The model under review builds one solid part; all positions refer to its coordinate system, in mm. Face numbers are marked on the shaded views. A direction names the side the tool comes from. Give positions to 0.01 mm unless a question says otherwise; leave off trailing zeros. Order: outer loops, then holes, each group sorted by start corner. A loop starts at its lowest first (then second) coordinate and runs counter-clockwise, first axis right, second up. Notation, with made-up numbers: (0.5, 16.25) - (25.5, 16.25) arc R9 cw to (25.5, 33.25) - close; hole circle Ø5 at (40.5, 50.5). An arc over 180 degrees is marked (long way). Write item = value, one per line. Start each with the question number.
1. We need section D-D, the plane z = 19.5. Give the boundary of the cut face in (x, y).
2. Wall thickness on probe 1 along X at (y, z) = (3.5, 29.5); probe 2 along Z at (x, y) = (6, 5.5); probe 3 along Z at (x, y) = (-6, 5.75): over which ranges is each line inside the solid? List them lowest first.
3. We need section B-B, the plane y = -3.5. Give the boundary of the cut face in (x, z) (3 decimals), and give its area (3 significant figures).
4. We need section C-C, the plane x = -5. Give the boundary of the cut face in (y, z).
5. Machinability: for the marked faces 1, 2 and 3, which of the approach directions +Z, -Z, +X, -X, +Y, -Y give a long, thin tool a straight path to every point of the face, cutting with its end or side? Answer none if there is none.
6. For P1, Ø6, axis at x = -13.5, z = 23.93, coming from the -Y side; P2, Ø4, axis at x = 1.86, z = 23.93, coming from the -Y side; P3, Ø1.4, axis at x = 2.5, z = 23.5, coming from the +Y side, all flat-tipped, find the tip position at first contact; note any pin that passes through.
7. We need section A-A, the plane y = 3. Give the boundary of the cut face in (x, z) (1 decimal), and give its area (3 significant figures).
8. Mouldability with a two-part tool opening along X and no side actions: class the marked faces 4, 5, 6 and 7 as pulls with the +X half, pulls with the -X half, needs draft (parallel to the pull), parting line crosses it, or undercut.
from build123d import *

# Parameters (mm, degrees)
F0_W          = 31.83
F0_H          = 15.82
F0_R          = 2.435
F1_DEPTH      = 2.5
F1_DEPTH_BACK = 9.6
F2_DEPTH      = 5
F3_R          = 3.215
F3_R_2        = 2.385
F4_DEPTH      = 8.4


with BuildPart() as f1:
    # F0 (on Front) → F1 (new body, two sides)
    with BuildSketch(Plane.XZ) as f1_sk:
        with Locations((-5.828721876, 24.0466938629)):
            Rectangle(F0_W, F0_H)
        with Locations((-17.828721876, 20.0516938629)):
            Circle(F0_R, mode=Mode.SUBTRACT)
        with Locations((-9.858721876, 20.0516938629)):
            Circle(F0_R, mode=Mode.SUBTRACT)
        with Locations((-1.798721876, 20.0516938629)):
            Circle(F0_R, mode=Mode.SUBTRACT)
        with Locations((6.171278124, 20.0516938629)):
            Circle(F0_R, mode=Mode.SUBTRACT)
        with Locations((-17.828721876, 28.0416938629)):
            Circle(F0_R, mode=Mode.SUBTRACT)
        with Locations((-9.858721876, 28.0416938629)):
            Circle(F0_R, mode=Mode.SUBTRACT)
        with Locations((-1.798721876, 28.0416938629)):
            Circle(F0_R, mode=Mode.SUBTRACT)
        with Locations((6.171278124, 28.0416938629)):
            Circle(F0_R, mode=Mode.SUBTRACT)
        with Locations((-1.798721876, 28.0416938629)):
            Circle(F0_R)
        with Locations((-9.858721876, 28.0416938629)):
            Circle(F0_R)
        with Locations((-17.828721876, 28.0416938629)):
            Circle(F0_R)
        with Locations((-17.828721876, 20.0516938629)):
            Circle(F0_R)
        with Locations((-9.858721876, 20.0516938629)):
            Circle(F0_R)
        with Locations((-1.798721876, 20.0516938629)):
            Circle(F0_R)
        with Locations((6.171278124, 20.0516938629)):
            Circle(F0_R)
        with Locations((6.171278124, 28.0416938629)):
            Circle(F0_R)
    extrude(amount=F1_DEPTH)
    extrude(f1_sk.sketch, amount=-F1_DEPTH_BACK)

    # F0 (on Front) → F2 (join)
    with BuildSketch(Plane.XZ):
        with Locations((-17.828721876, 28.0416938629)):
            Circle(F0_R)
        with Locations((-17.828721876, 20.0516938629)):
            Circle(F0_R)
        with Locations((-9.858721876, 28.0416938629)):
            Circle(F0_R)
        with Locations((-9.858721876, 20.0516938629)):
            Circle(F0_R)
        with Locations((-1.798721876, 28.0416938629)):
            Circle(F0_R)
        with Locations((-1.798721876, 20.0516938629)):
            Circle(F0_R)
        with Locations((6.171278124, 28.0416938629)):
            Circle(F0_R)
        with Locations((6.171278124, 20.0516938629)):
            Circle(F0_R)
    extrude(amount=F2_DEPTH)

    # F3 (on face) → F4 (cut)
    with BuildSketch(Plane(origin=(0, 9.6, 0), x_dir=(-1, 0, 0), z_dir=(0, 1, 0))):
        with BuildLine():
            Line((5.4793441668, 30.6818692116), (-8.7347330976, 30.6818692116))
            Line((-8.7347330976, 30.6818692116), (-8.7347330976, 17.3618692116))
            Line((-8.7347330976, 17.3618692116), (5.4793441668, 17.3618692116))
            Line((5.4793441668, 17.3618692116), (5.4793441668, 20.733492265))
            ThreePointArc((5.4793441668, 20.733492265), (2.6052669024, 23.9303652197), (5.4793441668, 27.1272381744))
            Line((5.4793441668, 27.1272381744), (5.4793441668, 30.6818692116))
        make_face()
        with Locations((-1.8597330976, 23.9303652197)):
            Circle(F3_R, mode=Mode.SUBTRACT)
        with BuildLine():
            Line((6.6202669024, 30.6818692116), (6.2793441668, 30.6818692116))
            Line((6.2793441668, 30.6818692116), (6.2793441668, 27.1124200692))
            ThreePointArc((6.2793441668, 27.1124200692), (8.2505095246, 26.0351563727), (9.0352669024, 23.9303652197))
            ThreePointArc((9.0352669024, 23.9303652197), (8.2505095246, 21.8255740668), (6.2793441668, 20.7483103702))
            Line((6.2793441668, 20.7483103702), (6.2793441668, 17.3618692116))
            Line((6.2793441668, 17.3618692116), (6.6202669024, 17.3618692116))
            Line((6.6202669024, 17.3618692116), (20.3752669024, 17.3618692116))
            Line((20.3752669024, 17.3618692116), (20.3752669024, 30.6818692116))
            Line((20.3752669024, 30.6818692116), (6.6202669024, 30.6818692116))
        make_face()
        with Locations((13.5002669024, 23.9303652197)):
            Circle(F3_R, mode=Mode.SUBTRACT)
        with Locations((-1.8597330976, 23.9303652197)):
            Circle(F3_R_2)
        with Locations((13.5002669024, 23.9303652197)):
            Circle(F3_R_2)
        with BuildLine():
            Line((5.4793441668, 21.5698575014), (5.4793441668, 26.290872938))
            ThreePointArc((5.4793441668, 26.290872938), (3.4352669024, 23.9303652197), (5.4793441668, 21.5698575014))
        make_face()
        with BuildLine():
            ThreePointArc((8.2052669024, 23.9303652197), (7.6618863359, 25.4458396874), (6.2793441668, 26.2707654131))
            Line((6.2793441668, 26.2707654131), (6.2793441668, 21.5899650263))
            ThreePointArc((6.2793441668, 21.5899650263), (7.6618863359, 22.414890752), (8.2052669024, 23.9303652197))
        make_face()
        with BuildLine():
            ThreePointArc((6.2793441668, 26.2707654131), (5.8801935351, 26.3146122285), (5.4793441668, 26.290872938))
            Line((5.4793441668, 26.290872938), (5.4793441668, 21.5698575014))
            ThreePointArc((5.4793441668, 21.5698575014), (5.8801935351, 21.546118211), (6.2793441668, 21.5899650263))
            Line((6.2793441668, 21.5899650263), (6.2793441668, 26.2707654131))
        make_face()
    extrude(amount=-F4_DEPTH, mode=Mode.SUBTRACT)


solid = f1.part
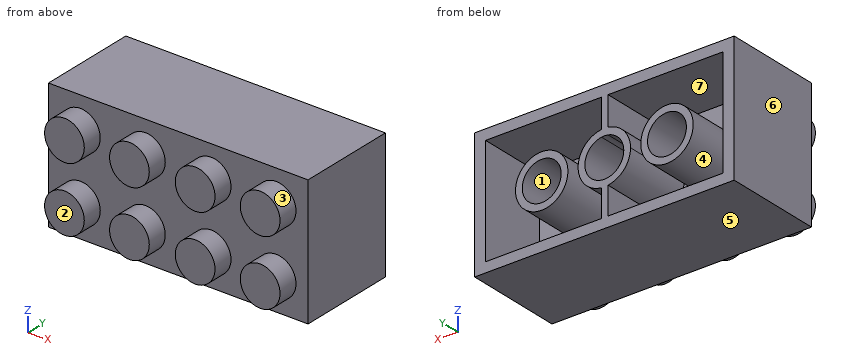
Model answer:
q1.outline = (-21.74, -2.5) - (-20.2, -2.5) - (-20.2, -5) - (-15.46, -5) - (-15.46, -2.5) - (-12.23, -2.5) - (-12.23, -5) - (-7.49, -5) - (-7.49, -2.5) - (-4.17, -2.5) - (-4.17, -5) - (0.57, -5) - (0.57, -2.5) - (3.8, -2.5) - (3.8, -5) - (8.54, -5) - (8.54, -2.5) - (10.09, -2.5) - (10.09, 9.6) - (8.73, 9.6) - (8.73, 1.2) - (-5.48, 1.2) - (-5.48, 9.6) - (-6.28, 9.6) - (-6.28, 1.2) - (-20.38, 1.2) - (-20.38, 9.6) - (-21.74, 9.6) - close
q2.probe_1 = -21.74 to -20.38, -6.28 to -5.48, 8.73 to 10.09
q2.probe_2 = 16.14 to 17.36, 30.68 to 31.96
q2.probe_3 = 16.14 to 21.55, 26.31 to 31.96
q3.outline = circle Ø4.87 at (-17.829, 20.052); circle Ø4.87 at (-17.829, 28.042); circle Ø4.87 at (-9.859, 20.052); circle Ø4.87 at (-9.859, 28.042); circle Ø4.87 at (-1.799, 20.052); circle Ø4.87 at (-1.799, 28.042); circle Ø4.87 at (6.171, 20.052); circle Ø4.87 at (6.171, 28.042)
q3.area = 149 mm2
q4.outline = (-2.5, 16.14) - (9.6, 16.14) - (9.6, 17.36) - (1.2, 17.36) - (1.2, 20.82) - (9.6, 20.82) - (9.6, 21.69) - (1.2, 21.69) - (1.2, 26.17) - (9.6, 26.17) - (9.6, 27.04) - (1.2, 27.04) - (1.2, 30.68) - (9.6, 30.68) - (9.6, 31.96) - (-2.5, 31.96) - close
q5.face_1 = +Y
q5.face_2 = +Z, -Z, +X, -X, -Y
q5.face_3 = -Y
q6.P1 = -5
q6.P2 = -2.5
q6.P3 = 1.2
q7.outline = (-21.7, 16.1) - (10.1, 16.1) - (10.1, 32) - (-21.7, 32) - close; circle Ø6.4 at (-13.5, 23.9); circle Ø6.4 at (1.9, 23.9); hole (-20.4, 17.4) - (-6.3, 17.4) - (-6.3, 20.7) arc R3.2 cw to (-6.3, 27.1) - (-6.3, 30.7) - (-20.4, 30.7) - close; hole circle Ø4.8 at (-13.5, 23.9); hole circle Ø4.8 at (-5.8, 23.9); hole (-5.5, 17.4) - (8.7, 17.4) - (8.7, 30.7) - (-5.5, 30.7) - (-5.5, 27.1) arc R3.2 cw to (-5.5, 20.7) - close; hole circle Ø4.8 at (1.9, 23.9)
q7.area = 165 mm2
q8.face_4 = undercut
q8.face_5 = needs draft
q8.face_6 = pulls with the -X half
q8.face_7 = undercut
